```python
from build123d import *

# Parameters (mm, degrees)
SKETCH1_W           = 110.49
SKETCH1_H           = 114.3
BOSS_EXTRUDE1_DEPTH = 2.54
SKETCH2_R           = 9.525
CUT_EXTRUDE1_DEPTH  = 2.54
SKETCH3_R           = 1.27
CUT_EXTRUDE2_DEPTH  = 159.993653018


with BuildPart() as part:
    # Sketch1 → Boss-Extrude1 (new body)
    with BuildSketch(Plane.XY):
        with Locations((55.245, -57.15)):
            Rectangle(SKETCH1_W, SKETCH1_H)
    extrude(amount=BOSS_EXTRUDE1_DEPTH)

    # Sketch2 → Cut-Extrude1 (cut)
    with BuildSketch(Plane.XY.offset(2.54)):
        with Locations((50.8, -57.15)):
            Circle(SKETCH2_R)
    extrude(amount=-CUT_EXTRUDE1_DEPTH, mode=Mode.SUBTRACT)

    # Sketch3 → Cut-Extrude2 (cut, through all)
    with BuildSketch(Plane.XY.offset(2.54)):
        with Locations((2.54, -4.826)):
            Circle(SKETCH3_R)
        with Locations(Location((2.54, -109.474, 0), (0, 0, 180))):
            Circle(SKETCH3_R)
        with Locations((105.41, -4.826)):
            Circle(SKETCH3_R)
        with Locations((105.41, -109.474)):
            Circle(SKETCH3_R)
    extrude(amount=-CUT_EXTRUDE2_DEPTH, mode=Mode.SUBTRACT)


solid = part.part
```
Geometry check sheet. Reference: the model listing, model coordinates, mm. Round coordinates to 2 decimals unless told otherwise and drop trailing zeros. Order: outer loops, then holes, each group sorted by start corner. A loop starts at its lowest first (then second) coordinate and runs counter-clockwise, first axis right, second up. Notation, with made-up numbers: (-22, -33.5) -> (8, -33.5) arc R20 cw to (8, -21.5) -> close; hole circle Ø8 at (8.5, -18.5). An arc over 180 degrees is marked (long way). Return JSON: item names as keys, results as strings. Group by question number.
Q1. Material ranges on probe 1 along Y at (x, z) = (105.41, 1.4); probe 2 along X at (y, z) = (-5, 0.2); probe 3 along Y at (x, z) = (50.8, 1.7) (3 decimals), recorded low to high. Write a range as from..to.
Q2. Section check B-B, the plane x = 50.8. Record the boundary of the cut face in (y, z) (3 decimals).
Q3. Release check for a two-part mould opening along Y. For faces 1 (the cylindrical face through (106.62, -4.44, 1.29)), 2 (the flat face through (54, -114.3, 1)), 3 (the flat face through (54, 0, 1)), 4 (the cylindrical face through (49.6, -47.7, 1.3)) record: released by +Y, released by -Y, zero draft, split by the parting line, or undercut.
Q4. Section check A-A, the plane y = -57.15. Record the boundary of the cut face in (x, z) (3 decimals).
Q5. Section check C-C, the plane z = 0.5. Record the boundary of the cut face in (x, y) (3 decimals).
Numbers:
{
 "1": {"probe 1": "-114.3..-110.74, -108.2..-6.1, -3.56..0", "probe 2": "0..1.28, 3.8..104.15, 106.67..110.49", "probe 3": "-114.3..-66.675, -47.625..0"},
 "2": {"outline": "(-114.3, 0) -> (-66.675, 0) -> (-66.675, 2.54) -> (-114.3, 2.54) -> close; (-47.625, 0) -> (0, 0) -> (0, 2.54) -> (-47.625, 2.54) -> close"},
 "3": {"face 1": "undercut", "face 2": "released by -Y", "face 3": "released by +Y", "face 4": "undercut"},
 "4": {"outline": "(0, 0) -> (41.275, 0) -> (41.275, 2.54) -> (0, 2.54) -> close; (60.325, 0) -> (110.49, 0) -> (110.49, 2.54) -> (60.325, 2.54) -> close"},
 "5": {"outline": "(0, -114.3) -> (110.49, -114.3) -> (110.49, 0) -> (0, 0) -> close; hole circle Ø2.54 at (2.54, -109.474); hole circle Ø2.54 at (2.54, -4.826); hole circle Ø19.05 at (50.8, -57.15); hole circle Ø2.54 at (105.41, -109.474); hole circle Ø2.54 at (105.41, -4.826)"}
}
